Geometry: final body of the model. Coordinates: model frame, mm. A direction names the side the tool comes from. Give positions to 0.01 mm unless a question says otherwise; leave off trailing zeros. Order: outer loops, then holes, each group sorted by start corner. A loop starts at its lowest first (then second) coordinate and runs counter-clockwise, first axis right, second up. Notation, with made-up numbers: M 31.5,-18 L 55.5,-18 A20 cw 55.5,14 Z; hole C 53.5,62.5 d10. An arc over 180 degrees is marked long. One line per item, written item: value. Start each with the question number.
```python
from build123d import *

# Parameters (mm, degrees)
SKETCH2_R          = 2
CUT_EXTRUDE1_DEPTH = 20
FILLET1_R          = 10


with BuildPart() as part:
    # Sketch1 → Revolve1 (revolve)
    with BuildSketch(Plane.XY, mode=Mode.PRIVATE) as revolve1_sk:
        Polygon((-170, 0), (-190, 0), (-70, 60), (-65, 60), (-65, 55), (-70, 55), (-70, 50), (0, 50), (0, 40), (-80, 40), (-80, 45), align=None)
    revolve(revolve1_sk.sketch.rotate(Axis((-170, 0, 0), (1, 0, 0)), 180), axis=Axis((-170, 0, 0), (1, 0, 0)))

    # Sketch2 → Cut-Extrude1 (cut)
    with BuildSketch(Plane(origin=(0, 0, 0), x_dir=(0, 0, -1), z_dir=(1, 0, 0))):
        with Locations(Location((0, 45, 0), (0, 0, 90))):
            Circle(SKETCH2_R)
        with Locations(Location((26.450336353, 36.405764747, 0), (0, 0, 90))):
            Circle(SKETCH2_R)
        with Locations(Location((42.797543233, 13.905764747, 0), (0, 0, 90))):
            Circle(SKETCH2_R)
        with Locations(Location((42.797543233, -13.905764747, 0), (0, 0, 90))):
            Circle(SKETCH2_R)
        with Locations(Location((26.450336353, -36.405764747, 0), (0, 0, 90))):
            Circle(SKETCH2_R)
        with Locations(Location((0, -45, 0), (0, 0, 90))):
            Circle(SKETCH2_R)
        with Locations(Location((-26.450336353, -36.405764747, 0), (0, 0, 90))):
            Circle(SKETCH2_R)
        with Locations(Location((-42.797543233, -13.905764747, 0), (0, 0, 90))):
            Circle(SKETCH2_R)
        with Locations(Location((-42.797543233, 13.905764747, 0), (0, 0, 90))):
            Circle(SKETCH2_R)
        with Locations(Location((-26.450336353, 36.405764747, 0), (0, 0, 90))):
            Circle(SKETCH2_R)
    extrude(amount=-CUT_EXTRUDE1_DEPTH, mode=Mode.SUBTRACT)

    # Fillet1
    fillet1_edges = [part.edges().sort_by_distance(p)[0] for p in [
        (-70, 60, 0),
    ]]
    fillet(fillet1_edges, radius=FILLET1_R)


solid = part.part
```
Q1. Mould query, pull axis Z, two halves, no side actions, for faces 3 (the face through (-66.301, 13.007, 58.573)), 4 (the face through (-136, -8, 15)), 5 (the face through (-20, -14, 43)), 6 (the face through (0, 34, 22)). Classes: +Z half, -Z half, draft (parallel to the pull), parting line (faces both ways), or undercut.
Q2. Ray query, line 1 along Z through (x, y) = (-57, 0); line 2 along Y through (x, z) = (-18.5, 43.5); line 3 along Y through (x, z) = (-99, -30). Return the intervals inside material, ascending. Write a range as [from, to].
Q3. Contact query for flat-ended pins moving along their axis: pin 1 (3 mm diameter, centred on y = 36.41, z = 26.45, fed in from +X); pin 2 (10 mm diameter, centred on x = -28, z = -43.5, fed in from -Y); pin 3 (4 mm diameter, centred on x = -113.5, y = -6, fed in from +Z); pin 4 (5 mm diameter, centred on x = -151, z = 23.5, fed in from +Y). Output: stop coordinate, or through.
Q4. Set-up query: faces 1 (the face through (-20, 14, -43)), 2 (the face through (-80, -30.2, 26.5)). Return all of +Z, -Z, +X, -X, +Y, -Y with unobstructed straight access to the full face (end or side cutting, diameter ignored); none if empty.
Q5. Section query C-C on x = -120. Return loops of the section in (y, z), and give its area (3 significant figures).
Q6. Section query B-B on x = -15.5. Give the number of separate pieces and of enclosed holes in the cut face, and give its area (3 significant figures).
Q7. Section query A-A on x = -91.5. Return loops of the section in (y, z), and give its area (3 significant figures).
Results below:
1. face 3: parting line
1. face 4: undercut
1. face 5: undercut
1. face 6: draft
2. line 1: [-50, -40], [40, 50]
2. line 2: [-24.65, -15.78], [-12.03, 12.03], [15.78, 24.65]
2. line 3: [-34.21, -18.98], [18.98, 34.21]
3. pin 1: x = -20
3. pin 2: y = -31.9
3. pin 3: z = 38.83
3. pin 4: through
4. face 1: +X
4. face 2: none
5. outline: C 0,0 d70; hole C 0,0 d50
5. area: 1,880 mm2
6. separate pieces: 1
6. enclosed holes: 11
6. area: 2,700 mm2
7. outline: C 0,0 d98.5; hole C 0,0 d78.5
7. area: 2,780 mm2
